Geometry: final body of the model. Coordinates: model frame, mm. Face numbers are marked on the shaded views. A direction names the side the tool comes from. Give positions to 0.01 mm unless a question says otherwise; leave off trailing zeros. Order: outer loops, then holes, each group sorted by start corner. A loop starts at its lowest first (then second) coordinate and runs counter-clockwise, first axis right, second up. Notation, with made-up numbers: (27.5, 67) - (77.5, 67) arc R8 cw to (77.5, 72) - close; hole circle Ø9 at (61.25, 39). An arc over 180 degrees is marked (long way). Put each result on its own line as item: value. Start each with the question number.
1. Section A-A on x = 17. Return the cut outline in (y, z).
2. Set-up query: the marked faces 5 and 6. Return all of +Z, -Z, +X, -X, +Y, -Y with unobstructed straight access to the full face (end or side cutting, diameter ignored); none if empty.
3. First-contact query: P1, Ø2, axis at x = -17.5, y = 19, coming from the +Z side; P2, Ø6, axis at x = -16.5, y = -22, coming from the -Z side (3 decimals); P3, Ø12, axis at x = -18.5, z = -22, coming from the +Y side. Flat tips, straight axial feed; report the tip coordinate or a pass-through.
4. Mould query, pull axis Y, two halves, no side actions, for the marked faces 1, 2, 3 and 4. Classes: pulls with the +Y half, pulls with the -Y half, needs draft (parallel to the pull), parting line crosses it, or undercut.
5. Ray query, line 1 along Z through (x, y) = (7.5, -4.5); line 2 along X through (y, z) = (45, -18.5); line 3 along X through (y, z) = (-13, -36.5) (3 decimals). Return the intervals inside material, ascending. Write a range as from..to.
6. Section B-B on y = 0. Count the separate pieces of the cut face and the enclosed holes in it, plus the area to 3 significant figures.
7. Section C-C on x = 1. Return the cut outline in (y, z) (1 decimal), plus the area to 3 significant figures.
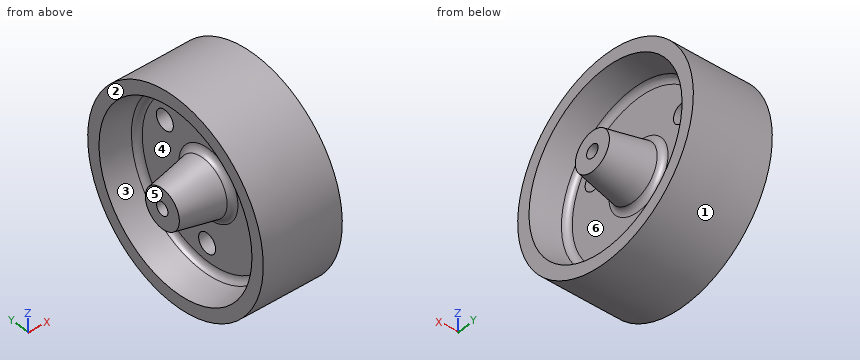
from build123d import *

# Parameters (mm, degrees)
F2_R     = 4.7625
F3_DEPTH = 50.801
F4_DEPTH = 50.801
F5_DEPTH = 50.801


with BuildPart() as f1:
    # F0 (on Front) → F1 (revolve)
    with BuildSketch(Plane.XZ):
        with BuildLine():
            Line((-25.4, -2.36029), (25.4, -2.336609))
            Line((25.4, -2.336609), (25.4, 4.013391))
            Line((25.4, 4.013391), (5.731009, 7.923037))
            ThreePointArc((5.731009, 7.923037), (3.895828, 9.022749), (3.175, 11.037114))
            Line((3.175, 11.037114), (3.175, 31.509514))
            ThreePointArc((3.175, 31.509514), (3.894639, 33.522429), (5.727331, 34.622857))
            Line((5.727331, 34.622857), (19.05, 37.287391))
            Line((19.05, 37.287391), (19.05, 43.637391))
            Line((19.05, 43.637391), (-19.05, 43.61371))
            Line((-19.05, 43.61371), (-19.05, 37.26371))
            Line((-19.05, 37.26371), (-5.727331, 34.599176))
            ThreePointArc((-5.727331, 34.599176), (-3.894639, 33.498747), (-3.175, 31.485832))
            Line((-3.175, 31.485832), (-3.175, 11.013432))
            ThreePointArc((-3.175, 11.013432), (-3.895828, 8.999068), (-5.731009, 7.899356))
            Line((-5.731009, 7.899356), (-25.4, 3.98971))
            Line((-25.4, 3.98971), (-25.4, -2.36029))
        make_face()
    revolve(axis=Axis((0.372264, 0, -5.53529), (1, 0, 0)))

    # F2 (on face) → F3 (cut, through all)
    with BuildSketch(Plane.YZ.offset(25.4)):
        with Locations((-25.092236, 8.136225)):
            Circle(F2_R)
    extrude(amount=-F3_DEPTH, mode=Mode.SUBTRACT)

    # F2 (on face) → F4 (cut, through all)
    with BuildSketch(Plane.YZ.offset(25.4)):
        with Locations((0.706239, -34.101561)):
            Circle(F2_R)
    extrude(amount=-F4_DEPTH, mode=Mode.SUBTRACT)

    # F2 (on face) → F5 (cut, through all)
    with BuildSketch(Plane.YZ.offset(25.4)):
        with Locations((24.385997, 9.359466)):
            Circle(F2_R)
    extrude(amount=-F5_DEPTH, mode=Mode.SUBTRACT)


solid = f1.part
Resolved:
1. outline: circle Ø98.34 at (0, -5.54); circle Ø22.44 at (0, -5.54); hole circle Ø84.83 at (0, -5.54); hole circle Ø6.39 at (0, -5.54)
2. face 5: +Z, -Z, -X, +Y, -Y
2. face 6: +X
3. P1: z = 40.2
3. P2: z = -50.865
3. P3: y = 48.02
4. face 1: parting line crosses it
4. face 2: needs draft
4. face 3: undercut
4. face 4: undercut
5. line 1: -54.49..-45.8, -17.85..6.77, 34.73..43.42
5. line 2: -19.05..19.05
5. line 3: -3.175..3.175
6. separate pieces: 3
6. enclosed holes: 0
6. area: 1,800 mm^2
7. outline: circle Ø98.3 at (0, -5.5); hole circle Ø9.5 at (-25.1, 8.1); hole circle Ø9.5 at (0.7, -34.1); hole circle Ø6.4 at (0, -5.5); hole circle Ø9.5 at (24.4, 9.4)
7. area: 7,350 mm^2
